```python
from build123d import *

# Parameters (mm, degrees)
SKETCH_R      = 2.5
EXTRUDE_DEPTH = 3


with BuildPart() as part:
    # Sketch → Extrude (new body)
    with BuildSketch(Plane.XY):
        with BuildLine():
            Line((-7.495407, 14.040454), (6.508806, 14.040454))
            Line((6.508806, 14.040454), (6.508806, 0))
            Line((6.508806, 0), (6.508806, -0.974619))
            Line((6.508806, -0.974619), (-3.635789, -0.974619))
            Line((-3.635789, 0), (-3.635789, -0.974619))
            ThreePointArc((-3.635789, 0), (-4.692641, 3.423621), (-7.495407, 5.6558))
            Line((-7.495407, 5.6558), (-7.495407, 14.040454))
        make_face()
        with Locations((0, 7.517769)):
            Circle(SKETCH_R, mode=Mode.SUBTRACT)
    extrude(amount=EXTRUDE_DEPTH)


solid = part.part
```
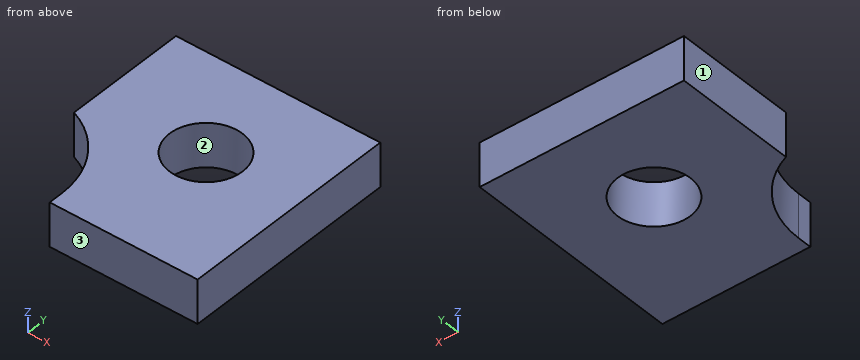
Geometry: final body of the model. Coordinates: model frame, mm. Face numbers are marked on the shaded views. Coordinates: 2 decimals unless noted, no trailing zeros. Order: outer loops, then holes, each group sorted by start corner. A loop starts at its lowest first (then second) coordinate and runs counter-clockwise, first axis right, second up. Notation, with made-up numbers: (22.5, 10.25) -> (57.5, 10.25) arc R3 ccw to (57.5, 14.25) -> close; hole circle Ø10 at (-21, -30.75). An arc over 180 degrees is marked (long way). Use CSV: the item, a comma, the result in double quotes.
1) Pin query (flat end, axial travel): pin 1 Ø8 at (x, y) = (-2.5, 1.5) entering from -Z; pin 2 Ø1 at (y, z) = (1, 1.5) entering from -X; pin 3 Ø0.8 at (y, z) = (-0.5, 1) entering from -X; pin 4 Ø3 at (x, y) = (0, 7.52) entering from -Z. Return the tip coordinate at first contact, or that it passes through.
Findings:
pin 1,"stops at z = 0"
pin 2,"stops at x = -3.82"
pin 3,"stops at x = -3.64"
pin 4,"passes through"
2) Mould query, pull axis Y, two halves, no side actions, for the marked faces 1, 2 and 3. Classes: +Y half, -Y half, draft (parallel to the pull), parting line (faces both ways), or undercut.
Findings:
face 1,"draft"
face 2,"undercut"
face 3,"-Y half"
3) Section B-B on y = 9.75. Output: boundary loops of the cut face in (x, z).
Findings:
outline,"(-7.5, 0) -> (-1.13, 0) -> (-1.13, 3) -> (-7.5, 3) -> close; (1.13, 0) -> (6.51, 0) -> (6.51, 3) -> (1.13, 3) -> close"
4) Section C-C on z = 0.5. Output: boundary loops of the cut face in (x, y), then the cut area to 3 significant figures.
Findings:
outline,"(-7.5, 5.66) arc R6.07 cw to (-3.64, 0) -> (-3.64, -0.97) -> (6.51, -0.97) -> (6.51, 14.04) -> (-7.5, 14.04) -> close; hole circle Ø5 at (0, 7.52)"
area,"171 mm^2"
5) Section A-A on x = 0. Output: boundary loops of the cut face in (y, z), then the cut area to 3 significant figures.
Findings:
outline,"(-0.97, 0) -> (5.02, 0) -> (5.02, 3) -> (-0.97, 3) -> close; (10.02, 0) -> (14.04, 0) -> (14.04, 3) -> (10.02, 3) -> close"
area,"30.0 mm^2"
6) Line query: line 1 (Y direction, x = 0, z = 2); line 2 (X direction, y = 6, z = 1.1); line 3 (X direction, y = 5.5, z = 0.7). Output: solid intervals per line, ascending.
Findings:
line 1,"y = -0.97 to 5.02, 10.02 to 14.04"
line 2,"x = -7.5 to -1.99, 1.99 to 6.51"
line 3,"x = -7.13 to -1.48, 1.48 to 6.51"
7) Section D-D on y = 4.5. Output: boundary loops of the cut face in (x, z), then the cut area to 3 significant figures.
Findings:
outline,"(-5.63, 0) -> (6.51, 0) -> (6.51, 3) -> (-5.63, 3) -> close"
area,"36.4 mm^2"
